from build123d import *

# Parameters (mm, degrees)
PAD_DEPTH = 10


with BuildPart() as part:
    # Sketch → Pad (new body)
    with BuildSketch(Plane.XZ):
        with BuildLine():
            Line((-3.1, -5.13712), (-3.1, -3.398529))
            ThreePointArc((3.1, -3.398529), (0, 4.6), (-3.1, -3.398529))
            Line((3.1, -5.13712), (3.1, -3.398529))
            ThreePointArc((-3.1, -5.13712), (0, -6), (3.1, -5.13712))
        make_face()
        with BuildLine():
            Line((1.5, 2.712932), (1.5, -2.712932))
            ThreePointArc((1.5, 2.712932), (-3.1, 0), (1.5, -2.712932))
        make_face(mode=Mode.SUBTRACT)
    extrude(amount=PAD_DEPTH)


solid = part.part
Source: CAD feature listing. Evaluate the final solid. Frame: model axes, mm. A direction names the side the tool comes from. Give positions to 0.01 mm unless a question says otherwise; leave off trailing zeros. Write each loop counter-clockwise with the first axis right and the second up, starting at its lowest first coordinate (ties: lowest second). Pieces come first, ordered by that corner, then holes. Notation, with made-up numbers: (75.5, 35.25) -> (119.5, 35.25) arc R15 ccw to (119.5, 54.25) -> close; hole circle Ø4 at (-37.75, 54.25). An arc over 180 degrees is marked (long way). Write item = value, one per line.
Q1. Cut plane D-D on z = -4. Return loops of the section in (x, y), then the cut area to 3 significant figures.
Here are the results:
outline = (-3.1, -10) -> (3.1, -10) -> (3.1, 0) -> (-3.1, 0) -> close
area = 62.0 mm²
Q2. Line query: line 1 (X direction, y = -4.5, z = 0); line 2 (Z direction, x = 0, y = -6.5); line 3 (Z direction, x = -1, y = -7.5). Output: solid intervals per line, ascending. Write a range as from..to.
Here are the results:
line_1 = -4.6..-3.1, 1.5..4.6
line_2 = -6..-3.1, 3.1..4.6
line_3 = -5.92..-2.93, 2.93..4.49
Q3. Cut plane C-C on y = -6.75. Return loops of the section in (x, z), then the cut area to 3 significant figures.
Here are the results:
outline = (-3.1, -5.14) arc R6 ccw to (3.1, -5.14) -> (3.1, -3.4) arc R4.6 ccw (long way) to (-3.1, -3.4) -> close; hole (1.5, -2.71) -> (1.5, 2.71) arc R3.1 ccw (long way) to start
area = 51.7 mm²
Q4. Mould query, pull axis Z, two halves, no side actions, for faces 3 (the face through (3.1, -5, -4)), 4 (the face through (1.5, -5, 0)), 5 (the face through (0.155, -4.93, 4.597)), 6 (the face through (-3.1, -4.9, 0.1)). Classes: +Z half, -Z half, draft (parallel to the pull), parting line (faces both ways), or undercut.
Here are the results:
face_3 = draft
face_4 = undercut
face_5 = parting line
face_6 = undercut
Q5. First-contact query: pin 1 (3 mm diameter, centred on y = -8, z = -2.5, fed in from -X); pin 2 (1.5 mm diameter, centred on x = -3, y = -3, fed in from +Z); pin 3 (6 mm diameter, centred on y = -4, z = -3.5, fed in from -X). Flat tips, straight axial feed; report the tip coordinate or a pass-through.
Here are the results:
pin_1 = -4.49
pin_2 = 4.01
pin_3 = -4.57
Q6. Cut plane B-B on z = 0. Return loops of the section in (x, y), then the cut area to 3 significant figures.
Here are the results:
outline = (-4.6, -10) -> (-3.1, -10) -> (-3.1, 0) -> (-4.6, 0) -> close; (1.5, -10) -> (4.6, -10) -> (4.6, 0) -> (1.5, 0) -> close
area = 46.0 mm²
Q7. Reachability of faces 1 (the face through (-3.1, -5, -4)), 2 (the face through (2, 0, -1)) from +Z, -Z, +X, -X, +Y, -Y: full face, straight path, thin tool, end or side. Return the list, or none.
Here are the results:
face_1 = -Z, -X, +Y, -Y
face_2 = +Z, -Z, +X, -X, +Y
Q8. Cut plane A-A on x = 0. Return loops of the section in (y, z), then the cut area to 3 significant figures.
Here are the results:
outline = (-10, -6) -> (0, -6) -> (0, -3.1) -> (-10, -3.1) -> close; (-10, 3.1) -> (0, 3.1) -> (0, 4.6) -> (-10, 4.6) -> close
area = 44.0 mm²
